from build123d import *

# Parameters (mm, degrees)
FILLET1_R      = 0.1
FILLET2_R      = 0.12
CHAMFER1_SIZE  = 0.2
EXTRUDE1_DEPTH = 1.3


with BuildPart() as part:
    # Sketch1 → Revolve1 (revolve)
    with BuildSketch(Plane.XY, mode=Mode.PRIVATE) as revolve1_sk:
        Polygon((3, 1.5), (3, 0), (4.279914881, 0), (19, 0), (19, 1.5), align=None)
        Polygon((0, 2.75), (0, 0), (3, 0), (3, 1.5), (3, 2.75), align=None)
    revolve(revolve1_sk.sketch.rotate(Axis((0, 0, 0), (1, 0, 0)), 90), axis=Axis((0, 0, 0), (1, 0, 0)))

    # Fillet1
    fillet1_edges = [part.edges().sort_by_distance(p)[0] for p in [
        (3, 0, -1.5),
    ]]
    fillet(fillet1_edges, radius=FILLET1_R)

    # Fillet2
    fillet2_edges = [part.edges().sort_by_distance(p)[0] for p in [
        (0, 0, -2.75),
    ]]
    fillet(fillet2_edges, radius=FILLET2_R)

    # Chamfer1
    chamfer1_edges = [part.edges().sort_by_distance(p)[0] for p in [
        (19, 0, -1.5),
    ]]
    chamfer(chamfer1_edges, length=CHAMFER1_SIZE)

    # Sketch2 → Extrude1 (cut)
    with BuildSketch(Plane.ZY):
        Polygon((0, 1.443375673), (-1.25, 0.721687836), (-1.25, -0.721687836), (0, -1.443375673), (1.25, -0.721687836), (1.25, 0.721687836), align=None)
    extrude(amount=-EXTRUDE1_DEPTH, mode=Mode.SUBTRACT)


solid = part.part
Model file for the job. Use its own axes, mm. A direction names the side the tool comes from. Coordinates: 2 decimals unless noted, no trailing zeros. Loops run counter-clockwise (first coordinate to the right, second up) from the corner with the lowest first, then second, coordinate; pieces in that order, holes last. Notation, with made-up numbers: (62.5, 16.25) -> (69.5, 16.25) arc R17 ccw to (69.5, 46.25) -> close; hole circle Ø6 at (-15.5, -34). An arc over 180 degrees is marked (long way). Use one line per item in the form item = value. Start each with the question number.
(1) Cut at B-B on x = 13. Give the cut face in (y, z), and give its area (3 significant figures).
(2) Cut at A-A on y = 0. Give the cut face in (x, z).
(3) Flat gauge pins, fed straight in: pin 1 (1 mm diameter, centred on y = -2, z = 1.5, fed in from -X); pin 2 (1.5 mm diameter, centred on x = 15.5, z = 1, fed in from -Y); pin 3 (1.5 mm diameter, centred on x = 15, y = 2, fed in from +Z). Where does each tip first touch, or does it go through?
(4) Tool access for faces 1 (the flat face through (0.641, 1.088, -0.616)), 2 (the cylindrical face through (10.84, -0.45, 1.43)), 3 (the flat face through (0, 1.1, 1.1)): list every direction of +Z, -Z, +X, -X, +Y, -Y with a clear straight run to the whole face (end or side of a thin tool).
(5) Pull direction Y, two halves, no side cores. Call faces 4 (the flat face through (0.641, -1.088, 0.616)), 5 (the flat face through (19, 0, 0)), 6 (the cylindrical face through (1.54, 2.685, -0.596)): pulls with the +Y half, pulls with the -Y half, needs draft (parallel to the pull), parting line crosses it, or undercut.
(6) Probe probe 1 along Y at (x, z) = (15.75, 0.05); probe 2 along X at (y, z) = (-1.85, -1.8). List the from-to ranges inside material, lowest first. Write a range as from..to.
Values:
q1.outline = circle Ø3 at (0, 0)
q1.area = 7.07 mm2
q2.outline = (0, -2.63) arc R0.12 ccw to (0.12, -2.75) -> (3, -2.75) -> (3, -1.6) arc R0.1 cw to (3.1, -1.5) -> (18.8, -1.5) -> (19, -1.3) -> (19, 1.3) -> (18.8, 1.5) -> (3.1, 1.5) arc R0.1 cw to (3, 1.6) -> (3, 2.75) -> (0.12, 2.75) arc R0.12 ccw to (0, 2.63) -> (0, 1.25) -> (1.3, 1.25) -> (1.3, -1.25) -> (0, -1.25) -> close
q3.pin_1 = 0
q3.pin_2 = -1.48
q3.pin_3 = 0.83
q4.face_1 = -X
q4.face_2 = +X
q4.face_3 = +Z, -Z, -X, +Y, -Y
q5.face_4 = undercut
q5.face_5 = needs draft
q5.face_6 = parting line crosses it
q6.probe_1 = -1.5..1.5
q6.probe_2 = 0..3
